The model under review builds one solid part; all positions refer to its coordinate system, in mm. A direction names the side the tool comes from. Coordinates: 2 decimals unless noted, no trailing zeros. Order: outer loops, then holes, each group sorted by start corner. A loop starts at its lowest first (then second) coordinate and runs counter-clockwise, first axis right, second up. Notation, with made-up numbers: (-0.5, 58) -> (54.5, 58) arc R21 ccw to (54.5, 95) -> close; hole circle Ø11 at (0.25, 38). An arc over 180 degrees is marked (long way). Put each result on its own line as item: value.
from build123d import *

# Parameters (mm, degrees)
F0_W      = 73
F0_H      = 73
F1_DEPTH  = 133.35
F2_R      = 36.5
F3_DEPTH  = 161.1
F4_R      = 27
F5_DEPTH  = 173.525
F6_R      = 9.45
F7_DEPTH  = 336
F8_R      = 57.112961
F8_R_2    = 13.335
F9_DEPTH  = 76
F10_R     = 82.497851
F10_R_2   = 13.335
F11_DEPTH = 76


with BuildPart() as f1:
    # F0 (on Front) → F1 (new body, symmetric)
    with BuildSketch(Plane.XZ):
        Rectangle(F0_W, F0_H)
    extrude(amount=F1_DEPTH, both=True)

    # F2 (on Right) → F3 (join)
    with BuildSketch(Plane.YZ):
        Circle(F2_R)
    extrude(amount=-F3_DEPTH)

    # F4 (on face) → F5 (cut)
    with BuildSketch(Plane(origin=(-161.1, 0, 0), x_dir=(0, -1, 0), z_dir=(-1, 0, 0))):
        Circle(F4_R)
    extrude(amount=-F5_DEPTH, mode=Mode.SUBTRACT)

    # F6 (on face) → F7 (cut)
    with BuildSketch(Plane.XZ.offset(133.35)):
        Circle(F6_R)
    extrude(amount=-F7_DEPTH, mode=Mode.SUBTRACT)

    # F8 (on face) → F9 (cut)
    with BuildSketch(Plane(origin=(0, 133.35, 0), x_dir=(-1, 0, 0), z_dir=(0, 1, 0))):
        Circle(F8_R)
        Circle(F8_R_2, mode=Mode.SUBTRACT)
    extrude(amount=-F9_DEPTH, mode=Mode.SUBTRACT)

    # F10 (on face) → F11 (cut)
    with BuildSketch(Plane.XZ.offset(133.35)):
        Circle(F10_R)
        Circle(F10_R_2, mode=Mode.SUBTRACT)
    extrude(amount=-F11_DEPTH, mode=Mode.SUBTRACT)


solid = f1.part
Item 1: Consider section D-D on y = -14. Write out the cut boundary in (x, z) (3 decimals).
Answers below:
outline: (-161.1, -33.708) -> (-36.5, -33.708) -> (-36.5, -36.5) -> (36.5, -36.5) -> (36.5, 36.5) -> (-36.5, 36.5) -> (-36.5, 33.708) -> (-161.1, 33.708) -> (-161.1, 23.087) -> (12.425, 23.087) -> (12.425, -23.087) -> (-161.1, -23.087) -> close
Item 2: Consider section B-B on x = 0. Write out the cut boundary in (y, z) (3 decimals).
Answers below:
outline: (-133.35, -13.335) -> (-57.35, -13.335) -> (-57.35, -36.5) -> (57.35, -36.5) -> (57.35, -13.335) -> (133.35, -13.335) -> (133.35, -9.45) -> (25.292, -9.45) arc R27 cw to (-25.292, -9.45) -> (-133.35, -9.45) -> close; (-133.35, 9.45) -> (-25.292, 9.45) arc R27 cw to (25.292, 9.45) -> (133.35, 9.45) -> (133.35, 13.335) -> (57.35, 13.335) -> (57.35, 36.5) -> (-57.35, 36.5) -> (-57.35, 13.335) -> (-133.35, 13.335) -> close
Item 3: For faces 1 (the flat face through (17, 57.35, 1)), 2 (the flat face through (12.425, 0, 0)), 3 (the cylindrical face through (9.014, 78.565, 2.839)), 4 (the flat face through (-36.5, 41, -1)), 5 (the cylindrical face through (-1.74, -95.88, 13.22)), list the 3-axis set-ups (+Z, -Z, +X, -X, +Y, -Y) from which the entire face can be reached by the end or side of a thin tool; tool diameter is ignored.
Answers below:
face 1: +Y
face 2: -X
face 3: +Y, -Y
face 4: -X, +Y
face 5: -Y
Item 4: For line 1 (Z direction, x = 0, y = -72) (3 decimals); line 2 (Z direction, x = 0, y = 57); line 3 (Y direction, x = -73, z = -1.5), list the stretches that pass through material, from the lowest coordinate up. Write a range as from..to.
Answers below:
line 1: -13.335..-9.45, 9.45..13.335
line 2: -36.5..-9.45, 9.45..36.5
line 3: -36.47..-26.96, 26.96..36.47
Item 5: Consider section A-A on z = 0. Write out the cut boundary in (x, y) (3 decimals), and give its area (3 significant figures).
Answers below:
outline: (-161.1, -36.5) -> (-36.5, -36.5) -> (-36.5, -57.35) -> (-13.335, -57.35) -> (-13.335, -133.35) -> (-9.45, -133.35) -> (-9.45, -27) -> (-161.1, -27) -> close; (-161.1, 27) -> (-9.45, 27) -> (-9.45, 133.35) -> (-13.335, 133.35) -> (-13.335, 57.35) -> (-36.5, 57.35) -> (-36.5, 36.5) -> (-161.1, 36.5) -> close; (9.45, -133.35) -> (13.335, -133.35) -> (13.335, -57.35) -> (36.5, -57.35) -> (36.5, 57.35) -> (13.335, 57.35) -> (13.335, 133.35) -> (9.45, 133.35) -> (9.45, 27) -> (12.425, 27) -> (12.425, -27) -> (9.45, -27) -> close
area: 8,130 mm^2
Item 6: Consider section C-C on y = -42. Write out the cut boundary in (x, z), and give its area (3 significant figures).
Answers below:
outline: (-36.5, -36.5) -> (36.5, -36.5) -> (36.5, 36.5) -> (-36.5, 36.5) -> close; hole circle Ø18.9 at (0, 0)
area: 5,050 mm^2
Item 7: Mouldability with a two-part tool opening along Z and no side actions: class faces 6 (the flat face through (-36.5, -42, -1)), 7 (the cylindrical face through (-75.55, 5.85, -26.36)), 8 (the cylindrical face through (-97.928, -7.912, -35.632)) as +Z half, -Z half, draft (parallel to the pull), parting line (faces both ways), or undercut.
Answers below:
face 6: draft
face 7: undercut
face 8: parting line
Item 8: For pin 1 Ø4 at (y, z) = (-42, -8.5) entering from -X; pin 2 Ø10 at (y, z) = (-95, -10) entering from -X; pin 3 Ø15 at (x, z) = (0, 0) entering from +Y; pin 4 Ø2 at (x, z) = (-17.5, 20.5) entering from -Y, all flat-tipped, find the tip position at first contact; note any pin that passes through.
Answers below:
pin 1: x = -36.5
pin 2: x = -12.36
pin 3: through
pin 4: y = -57.35
